Source: CAD feature listing. Evaluate the final solid. Frame: model axes, mm. Face numbers are marked on the shaded views. Round coordinates to 2 decimals unless told otherwise and drop trailing zeros. Write each loop counter-clockwise with the first axis right and the second up, starting at its lowest first coordinate (ties: lowest second). Pieces come first, ordered by that corner, then holes. Notation, with made-up numbers: M -40,51 L 11,51 A25 ccw 11,64 Z; hole C -32,-32 d6. An arc over 180 degrees is marked long. Use a Markdown table: item, result.
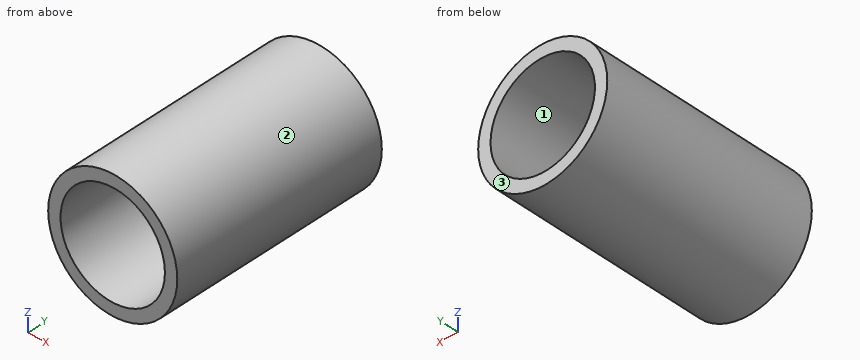
```python
from build123d import *

# Parameters (mm, degrees)
F0_R     = 73.3332365525
F0_R_2   = 59.319487814
F1_DEPTH = 254
F2_T     = -2.54


with BuildPart() as f1:
    # F0 (on Front) → F1 (new body)
    with BuildSketch(Plane.XZ):
        Circle(F0_R)
        Circle(F0_R_2, mode=Mode.SUBTRACT)
    extrude(amount=-F1_DEPTH)

    # F2 (hollow: no face is removed)
    offset(amount=F2_T, mode=Mode.SUBTRACT)


solid = f1.part
```
Q1. First-contact query: pin 1 Ø12 at (y, z) = (137.5, 38.5) entering from +X; pin 2 Ø12 at (y, z) = (43.5, -55) entering from +X; pin 3 Ø2 at (y, z) = (71, -18) entering from +X. Flat tips, straight axial feed; report the tip coordinate or a pass-through.
Results are:
| item | result |
|---|---|
| pin 1 | x = 65.74 |
| pin 2 | x = 54.56 |
| pin 3 | x = 71.34 |
Q2. Mould query, pull axis X, two halves, no side actions, for the marked faces 1, 2 and 3. Classes: +X half, -X half, draft (parallel to the pull), parting line (faces both ways), or undercut.
Results are:
| item | result |
|---|---|
| face 1 | undercut |
| face 2 | parting line |
| face 3 | draft |
Q3. Section B-B on z = 0. Return loops of the section in (x, y).
Results are:
| item | result |
|---|---|
| outline | M -73.33,0 L -59.32,0 L -59.32,254 L -73.33,254 Z; M 59.32,0 L 73.33,0 L 73.33,254 L 59.32,254 Z; hole M -70.79,2.54 L -61.86,2.54 L -61.86,251.46 L -70.79,251.46 Z; hole M 61.86,2.54 L 70.79,2.54 L 70.79,251.46 L 61.86,251.46 Z |
Q4. Line query: L1, parallel to Z at x = 0, y = 108; L2, parallel to Y at x = 37, z = 54; L3, parallel to Z at x = 10, y = 128.5. Output: solid intervals per line, ascending.
Results are:
| item | result |
|---|---|
| L1 | -73.33 to -70.79, -61.86 to -59.32, 59.32 to 61.86, 70.79 to 73.33 |
| L2 | 0 to 2.54, 251.46 to 254 |
| L3 | -72.65 to -70.08, -61.05 to -58.47, 58.47 to 61.05, 70.08 to 72.65 |
Q5. Section C-C on y = 58. Return loops of the section in (x, z).
Results are:
| item | result |
|---|---|
| outline | C 0,0 d146.67; C 0,0 d123.72; hole C 0,0 d141.59; hole C 0,0 d118.64 |
Q6. Section A-A on x = 0. Return loops of the section in (y, z).
Results are:
| item | result |
|---|---|
| outline | M 0,-73.33 L 254,-73.33 L 254,-59.32 L 0,-59.32 Z; M 0,59.32 L 254,59.32 L 254,73.33 L 0,73.33 Z; hole M 2.54,-70.79 L 251.46,-70.79 L 251.46,-61.86 L 2.54,-61.86 Z; hole M 2.54,61.86 L 251.46,61.86 L 251.46,70.79 L 2.54,70.79 Z |
